The model under review builds one solid part; all positions refer to its coordinate system, in mm. A direction names the side the tool comes from. Round coordinates to 2 decimals unless told otherwise and drop trailing zeros. Order: outer loops, then holes, each group sorted by start corner. A loop starts at its lowest first (then second) coordinate and runs counter-clockwise, first axis right, second up. Notation, with made-up numbers: (70, 58.5) -> (118, 58.5) arc R21 cw to (118, 91.5) -> close; hole circle Ø2 at (80, 76.5). An arc over 180 degrees is marked (long way). Return JSON: item names as keys, results as strings. Group by question number.
from build123d import *

# Parameters (mm, degrees)
F1_DEPTH = 2.286
F0_R     = 3.609475
F0_R_2   = 3.720562
F2_DEPTH = 14.986
F3_DEPTH = 21.59


with BuildPart() as f1:
    # F0 (on Top) → F1 (new body)
    with BuildSketch(Plane.XY):
        Polygon((36.545925, 46.772763), (27.516532, 56.097239), (-27.823025, 56.097239), (-35.342764, 48.298985), (-36.545925, -47.97592), (-27.516532, -56.097239), (27.823025, -56.097239), (36.545925, -47.97592), align=None)
    extrude(amount=F1_DEPTH)

    # F0 (on Top) → F2 (join)
    with BuildSketch(Plane.XY):
        Polygon((-35.342764, 48.298985), (-27.823025, 56.097239), (-36.245134, 64.218551), (-43.653179, 56.312592), align=None)
        with Locations((-35.342764, 56.097239)):
            Circle(F0_R, mode=Mode.SUBTRACT)
        Polygon((-27.516532, -56.097239), (-36.545925, -47.97592), (-44.083779, -56.356608), (-35.342764, -64.218551), align=None)
        with Locations((-35.342764, -56.097239)):
            Circle(F0_R_2, mode=Mode.SUBTRACT)
    extrude(amount=F2_DEPTH)

    # F0 (on Top) → F3 (join)
    with BuildSketch(Plane.XY):
        with Locations((-35.342764, 56.097239)):
            Circle(F0_R)
        with Locations((-35.342764, -56.097239)):
            Circle(F0_R_2)
    extrude(amount=F3_DEPTH)


solid = f1.part
Item 1: For faces 5 (the face through (-31.64, 52.14, 8.55)), 6 (the face through (-39.556, 52.362, 7.388)), 7 (the face through (-31.975, 60.101, 7.388)), 8 (the face through (-35, 56, 21.59)), 9 (the face through (-39, 55, 14.986)), list the 3-axis set-ups (+Z, -Z, +X, -X, +Y, -Y) from which the entire face can be reached by the end or side of a thin tool; tool diameter is ignored.
Item 2: The part is to be moulded in two halves that separate along Y. For faces 1 (the face through (32.123, -52.093, 1.127)), 2 (the face through (-39.9, 60.32, 7.39)), 3 (the face through (-4, 1, 0)), 4 (the face through (-31.97, -52.09, 8.55)), say which applies: +Y half, -Y half, draft (parallel to the pull), parting line (faces both ways), or undercut.
Item 3: Insertion check: pin 1 Ø10 at (x, y) = (-16, 4.5) entering from +Z; pin 2 Ø1 at (x, z) = (-12.5, 2) entering from +Y; pin 3 Ø18 at (x, y) = (-39.5, -56) entering from +Z; pin 4 Ø2.5 at (x, z) = (-5, 1.5) entering from -Y. Each pin has a flat end and moves straight along its axis. Give the tip position at first contact, or say it passes through.
Item 4: Consider section C-C on z = 16.25. State the section outline as (x, y) points.
Item 5: Consider section D-D on y = -40.5. State the section outline as (x, z) points.
Item 6: Wall thickness on line 1 along Z through (x, y) = (22.5, 37.5); line 2 along X through (y, z) = (-23.5, 2); line 3 along X through (y, z) = (58, 9.75): over which ranges is each line inside the solid? List them lowest first.
Item 7: Consider section A-A on z = 8. State the section outline as (x, y) points.
Item 8: Consider section B-B on x = -11.5. State the section outline as (y, z) points.
Values:
{
 "1": {"face 5": "+Z, +X", "face 6": "+Z, -Z, -X", "face 7": "+Z, -Z, +X, +Y", "face 8": "+Z, +X, -X, +Y, -Y", "face 9": "+Z"},
 "2": {"face 1": "-Y half", "face 2": "+Y half", "face 3": "draft", "face 4": "undercut"},
 "3": {"pin 1": "z = 2.29", "pin 2": "y = 56.1", "pin 3": "z = 21.59", "pin 4": "y = -56.1"},
 "4": {"outline": "circle Ø7.44 at (-35.34, -56.1); circle Ø7.22 at (-35.34, 56.1)"},
 "5": {"outline": "(-36.45, 0) -> (36.55, 0) -> (36.55, 2.29) -> (-36.45, 2.29) -> close"},
 "6": {"line 1": "0 to 2.29", "line 2": "-36.24 to 36.55", "line 3": "-42.07 to -29.8"},
 "7": {"outline": "(-44.08, -56.36) -> (-35.34, -64.22) -> (-27.52, -56.1) -> (-36.55, -47.98) -> close; (-43.65, 56.31) -> (-35.34, 48.3) -> (-27.82, 56.1) -> (-36.25, 64.22) -> close"},
 "8": {"outline": "(-56.1, 0) -> (56.1, 0) -> (56.1, 2.29) -> (-56.1, 2.29) -> close"}
}
